Can you work these out from the drawing? Everything is in mm from the part's minimum corner. Coordinates: 2 decimals unless noted, no trailing zeros. Order: outer loops, then holes, each group sorted by start corner. A loop starts at its lowest first (then second) coordinate and runs counter-clockwise, first axis right, second up. Notation, with made-up numbers: (-28.75, 43) -> (-3.75, 43) arc R13 ccw to (-3.75, 51) -> close; hole circle Ø10 at (66, 86.25). An arc over 180 degrees is marked (long way). Put each result on its own line as item: value. Start each with the question number.
Q1. If we section it at C-C (z = 1.65): Count the separate pieces of the cut face and the enclosed holes in it, and give its area (3 significant figures).
Q2. If we section it at A-A (x = 5): Please give me the cut outline in (y, z).
Q3. Please list where these lines run through material, in increasing order: line 1 along Y through (x, z) = (22.5, 3.9); line 2 along Y through (x, z) = (4.5, 4.4); line 3 along X through (y, z) = (18.5, 0.6).
Q4. If we section it at B-B (y = 17.5): Please give me the cut outline in (x, z).
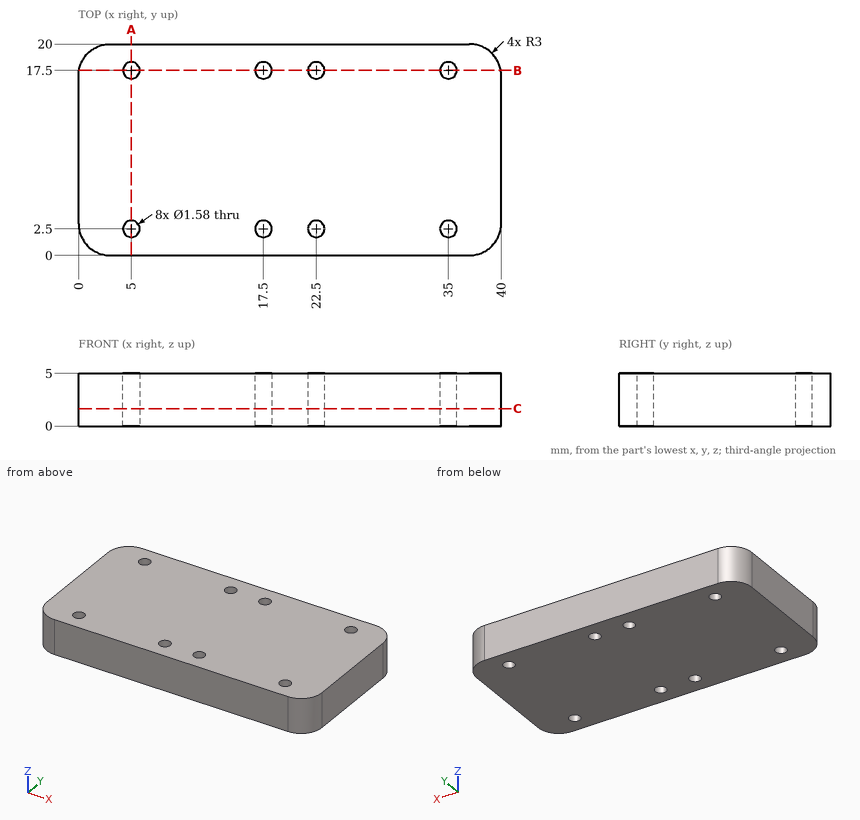
The answers:
1. separate pieces: 1
1. enclosed holes: 8
1. area: 777 mm^2
2. outline: (0, 0) -> (1.71, 0) -> (1.71, 5) -> (0, 5) -> close; (3.29, 0) -> (16.71, 0) -> (16.71, 5) -> (3.29, 5) -> close; (18.29, 0) -> (20, 0) -> (20, 5) -> (18.29, 5) -> close
3. line 1: 0 to 1.71, 3.29 to 16.71, 18.29 to 20
3. line 2: 0 to 1.89, 3.11 to 16.89, 18.11 to 20
3. line 3: 0.4 to 39.6
4. outline: (0.04, 0) -> (4.21, 0) -> (4.21, 5) -> (0.04, 5) -> close; (5.79, 0) -> (16.71, 0) -> (16.71, 5) -> (5.79, 5) -> close; (18.29, 0) -> (21.71, 0) -> (21.71, 5) -> (18.29, 5) -> close; (23.29, 0) -> (34.21, 0) -> (34.21, 5) -> (23.29, 5) -> close; (35.79, 0) -> (39.96, 0) -> (39.96, 5) -> (35.79, 5) -> close
